Build history of the part. All positions in model axes, mm. A direction names the side the tool comes from. Round coordinates to 2 decimals unless told otherwise and drop trailing zeros. Write each loop counter-clockwise with the first axis right and the second up, starting at its lowest first coordinate (ties: lowest second). Pieces come first, ordered by that corner, then holes. Notation, with made-up numbers: M 11,22 L 17,22 A28 ccw 17,61 Z; hole C 76.25,56 d1. An arc over 180 degrees is marked long. One line per item, written item: value. Start each with the question number.
```python
from build123d import *

# Parameters (mm, degrees)
SKETCH1_W           = 32.5
SKETCH1_H           = 12
BOSS_EXTRUDE1_DEPTH = 2
SKETCH2_W           = 2
SKETCH2_H           = 12
BOSS_EXTRUDE2_DEPTH = 17
SKETCH3_W           = 12
SKETCH3_H           = 2
BOSS_EXTRUDE3_DEPTH = 3
SKETCH4_W           = 12
SKETCH4_H           = 2
BOSS_EXTRUDE4_DEPTH = 3
SKETCH5_W           = 32.5
SKETCH5_H           = 2
BOSS_EXTRUDE6_DEPTH = 10
SKETCH7_W           = 32.5
SKETCH7_H           = 2
BOSS_EXTRUDE7_DEPTH = 10
FILLET1_R           = 5
SKETCH8_R           = 1
CUT_EXTRUDE1_DEPTH  = 10


with BuildPart() as part:
    # Sketch1 → Boss-Extrude1 (new body)
    with BuildSketch(Plane(origin=(0, 0, 0), x_dir=(1, 0, 0), z_dir=(0, 1, 0))):
        with Locations((16.25, 6)):
            Rectangle(SKETCH1_W, SKETCH1_H)
    extrude(amount=BOSS_EXTRUDE1_DEPTH)

    # Sketch2 → Boss-Extrude2 (add)
    with BuildSketch(Plane(origin=(0, 2, 0), x_dir=(1, 0, 0), z_dir=(0, 1, 0))):
        with Locations((1, 6)):
            Rectangle(SKETCH2_W, SKETCH2_H)
        with Locations((31.5, 6)):
            Rectangle(SKETCH2_W, SKETCH2_H)
    extrude(amount=BOSS_EXTRUDE2_DEPTH)

    # Sketch3 → Boss-Extrude3 (add)
    with BuildSketch(Plane(origin=(2, 0, 0), x_dir=(0, 0, -1), z_dir=(1, 0, 0))):
        with Locations((6, 18)):
            Rectangle(SKETCH3_W, SKETCH3_H)
    extrude(amount=BOSS_EXTRUDE3_DEPTH)

    # Sketch4 → Boss-Extrude4 (add)
    with BuildSketch(Plane.ZY.offset(-30.5)):
        with Locations((-6, 18)):
            Rectangle(SKETCH4_W, SKETCH4_H)
    extrude(amount=BOSS_EXTRUDE4_DEPTH)

    # Sketch5 → Boss-Extrude6 (add)
    with BuildSketch(Plane(origin=(0, 0, -12), x_dir=(-1, 0, 0), z_dir=(0, 0, -1))):
        with Locations((-16.25, 1)):
            Rectangle(SKETCH5_W, SKETCH5_H)
    extrude(amount=BOSS_EXTRUDE6_DEPTH)

    # Sketch7 → Boss-Extrude7 (add)
    with BuildSketch(Plane.XY):
        with Locations((16.25, 1)):
            Rectangle(SKETCH7_W, SKETCH7_H)
    extrude(amount=BOSS_EXTRUDE7_DEPTH)

    # Fillet1
    fillet1_edges = [part.edges().sort_by_distance(p)[0] for p in [
        (32.5, 1, 10),
        (0, 1, 10),
        (32.5, 1, -22),
        (0, 1, -22),
    ]]
    fillet(fillet1_edges, radius=FILLET1_R)

    # Sketch8 → Cut-Extrude1 (cut)
    with BuildSketch(Plane(origin=(0, 19, 0), x_dir=(1, 0, 0), z_dir=(0, 1, 0))):
        with Locations(Location((2.5, 5.75, 0), (0, 0, 270))):
            Circle(SKETCH8_R)
        with Locations(Location((30, 5.75, 0), (0, 0, 270))):
            Circle(SKETCH8_R)
    extrude(amount=-CUT_EXTRUDE1_DEPTH, mode=Mode.SUBTRACT)


solid = part.part
```
Item 1: Cut at B-B, the plane z = -5.75. Write the cut outline in (x, y), plus the area to 3 significant figures.
Item 2: Cut at A-A, the plane y = 16.25. Write the cut outline in (x, z), plus the area to 3 significant figures.
Item 3: Drop flat-ended pins along their axis: pin 1 (2.5 mm diameter, centred on x = 31, y = 7, fed in from +Z); pin 2 (4 mm diameter, centred on x = 1.5, y = 7.5, fed in from -Z); pin 3 (1.2 mm diameter, centred on x = 2.5, z = -5.75, fed in from +Y). Give the stop position or say it passes through.
Item 4: Cut at D-D, the plane x = 4.5. Write the cut outline in (y, z).
Item 5: Cut at C-C, the plane x = 30. Write the cut outline in (y, z), plus the area to 3 significant figures.
Item 6: Which spindle directions (+Z, -Z, +X, -X, +Y, -Y) get a long thin tool onto all of the face, cutting with end or side? Do faces 1 (the flat face through (5, 18, -6)), 2 (the cylindrical face through (1.524, 15.181, -5.967)), 3 (the flat face through (31, 10, -12)), 4 (the flat face through (31, 10, 0)), 5 (the flat face through (4, 17, -6)). Say none if no direction does.
Item 7: Drill centre lines: line 1 (X direction, y = 7.25, z = -9); line 2 (X direction, y = 12.5, z = -5.75); line 3 (Y direction, x = 28.5, z = -1). Where is each one in solid material? Low to high.
Item 8: Two-plate mould, pull along Y, no slides. Class faces 6 (the flat face through (31.1, 19, -6.1)), 7 (the flat face through (28.7, 17, -6.1)), 8 (the cylindrical face through (1, 1, 8)): pulls with the +Y half, pulls with the -Y half, needs draft (parallel to the pull), parting line crosses it, or undercut.
Computed values:
1. outline: M 0,0 L 32.5,0 L 32.5,19 L 31,19 L 31,9 L 30.5,9 L 30.5,2 L 2,2 L 2,9 L 1.5,9 L 1.5,19 L 0,19 Z; M 3.5,17 L 5,17 L 5,19 L 3.5,19 Z; M 27.5,17 L 29,17 L 29,19 L 27.5,19 Z
1. area: 129 mm2
2. outline: M 0,-12 L 2,-12 L 2,-6.62 A1 cw 2,-4.88 L 2,0 L 0,0 Z; M 30.5,-12 L 32.5,-12 L 32.5,0 L 30.5,0 L 30.5,-4.88 A1 cw 30.5,-6.62 Z
2. area: 46.8 mm2
3. pin 1: stops at z = 0
3. pin 2: stops at z = -12
3. pin 3: stops at y = 9
4. outline: M 0,-21.97 L 2,-21.97 L 2,9.97 L 0,9.97 Z; M 17,-12 L 19,-12 L 19,0 L 17,0 Z
5. outline: M 0,-21.33 L 2,-21.33 L 2,9.33 L 0,9.33 Z; M 17,-12 L 19,-12 L 19,-6.75 L 17,-6.75 Z; M 17,-4.75 L 19,-4.75 L 19,0 L 17,0 Z
5. area: 81.3 mm2
6. face 1: +Z, -Z, +Y
6. face 2: +Y
6. face 3: -Z, +X, -X, +Y
6. face 4: +Z, +X, -X, +Y
6. face 5: +Z, -Z
7. line 1: x = 0 to 2, 30.5 to 32.5
7. line 2: x = 0 to 1.5, 31 to 32.5
7. line 3: y = 0 to 2, 17 to 19
8. face 6: pulls with the +Y half
8. face 7: undercut
8. face 8: needs draft
